Read the model definition and answer for the solid it produces. Units are mm, in the model's axes. A direction names the side the tool comes from. Coordinates: 2 decimals unless noted, no trailing zeros.
Item 1: Each of these flat-tipped pins is pushed along its axis until it touches: P1, Ø5.5, axis at y = 57.5, z = 11.5, coming from the -X side; P2, Ø3, axis at x = 3, z = 5, coming from the -Y side; P3, Ø4, axis at x = 13, z = 15, coming from the -Y side (3 decimals); P4, Ø6, axis at x = 2, z = 3.5, coming from the +Y side. Where does it stop, or does it pass through?
Item 2: Straight lines are drawn through the part: probe 1 along Y at (x, z) = (12.5, 12) (3 decimals); probe 2 along Y at (x, z) = (2.25, 16.25); probe 3 along X at (y, z) = (19.5, 2.75) (3 decimals). For each, find the intervals that lie inside material, in ascending order.
Item 3: A tool of negligible diameter and unlimited length cuts with its end or side. For faces 1 (the face through (12.7, 56, 9)), 2 (the face through (8.026, 48.078, 0.477)), 3 (the face through (13.18, 56.28, 18.6)), 4 (the face through (13.18, 56.43, 0.45)), 5 (the face through (3.175, 24, 9)), from which of +Z, -Z, +X, -X, +Y, -Y can it reach the whole face along a straight path? Write none if from no direction.
Autodesk Inventor part; units mm, degrees
ref_plane "YZ Plane" through (0, 0, 0) normal (1, 0, 0) x (0, 1, 0)
ref_plane "XZ Plane" through (0, 0, 0) normal (0, 1, 0) x (-1, 0, 0)
ref_plane "XY Plane" through (0, 0, 0) normal (0, 0, 1) x (1, 0, 0)
sketch "Sketch1" plane through (0, 0, 0) normal (0, 0, 1) x (1, 0, 0)
  line L0 (0, 0) -> (0, 50.8)
  line L1 (0, 50.8) -> (12.7, 50.8)
  line L2 (12.7, 50.8) -> (12.7, 63.5)
  line L3 (12.7, 63.5) -> (15.875, 63.5)
  line L4 (15.875, 63.5) -> (15.875, 47.625)
  line L5 (15.875, 47.625) -> (3.175, 47.625)
  line L6 (3.175, 47.625) -> (3.175, 0)
  line L7 (3.175, 0) -> (0, 0)
extrude "Extrusion1" add sketch "Sketch1" along normal blind 19.05
fillet "Fillet1" radius 1.5875 1 edges at (15.875, 55.5625, 19.05)
fillet "Fillet2" radius 1.5875 1 edges at (15.875, 55.5625, 0)
fillet "Fillet3" radius 1.5875 5 edges at (15.875, 63.5, 9.525) (15.41, 63.5, 18.585) (13.4938, 63.5, 19.05) (15.41, 63.5, 0.465) (13.4938, 63.5, 0)
fillet "Fillet4" radius 1.5875 5 edges at (12.7, 63.5, 9.525) (12.7, 63.035, 18.585) (12.7, 56.3563, 19.05) (12.7, 63.035, 0.465) (12.7, 56.3563, 0)
fillet "Fillet5" radius 1.5875 1 edges at (0, 50.8, 9.525)
fillet "Fillet6" radius 1.5875 1 edges at (3.175, 23.8125, 19.05)
fillet "Fillet7" radius 1.5875 5 edges at (8.7312, 47.625, 19.05) (15.41, 47.625, 18.585) (15.875, 47.625, 9.525) (15.41, 47.625, 0.465) (8.7312, 47.625, 0)
fillet "Fillet8" radius 1.5875 1 edges at (3.175, 23.8125, 0)
properties part number "Z-Clip"
Established:
1. P1: stops at x = 12.7
1. P2: stops at y = 0
1. P3: stops at y = 47.625
1. P4: stops at y = 50.8
2. probe 1: y = 47.625 to 50.8
2. probe 2: y = 0 to 50.8
2. probe 3: x = 0 to 3.175
3. face 1: +Z, -Z, -X, +Y
3. face 2: -Z, +X, -Y
3. face 3: +Z, -X, +Y
3. face 4: -Z, -X, +Y
3. face 5: +Z, -Z, +X, -Y
